Could you check a few things on this model? Use its own coordinates, in mm. A direction names the side the tool comes from. Give positions to 0.01 mm unless a question says otherwise; leave off trailing zeros. Write each loop counter-clockwise with the first axis right and the second up, starting at its lowest first coordinate (ties: lowest second). Pieces come first, ordered by that corner, then holes. Notation, with made-up numbers: (-3, 50) -> (14, 50) arc R26 cw to (14, 89) -> close; hole circle Ø11 at (62, 1). An arc over 180 degrees is marked (long way). One line per question, with ' | ' between items.
Autodesk Inventor part; units mm, degrees
ref_plane "YZ Plane" through (0, 0, 0) normal (1, 0, 0) x (0, 1, 0)
ref_plane "XZ Plane" through (0, 0, 0) normal (0, 1, 0) x (-1, 0, 0)
ref_plane "XY Plane" through (0, 0, 0) normal (0, 0, 1) x (1, 0, 0)
sketch "Sketch1" plane through (0, 0, 0) normal (0, 0, 1) x (1, 0, 0)
  line L0 (0, 3) -> (0, 18)
  line L1 (0, 18) -> (4, 18)
  line L2 (4, 18) -> (4, 15)
  line L3 (4, 15) -> (94, 15)
  line L4 (94, 15) -> (94, 18)
  line L5 (94, 18) -> (98, 18)
  line L6 (98, 18) -> (98, 12)
  line L7 (98, 12) -> (3, 12)
  line L8 (3, 12) -> (3, 3)
  line L9 (3, 0) -> (0, 0) construction
  line L10 (0, 3) -> (3, 3)
  dimension "d0" = 18
  dimension "d1" = 4
  dimension "d2" = 3
  dimension "d3" = 90
  dimension "d4" = 4
  dimension "d5" = 6
  dimension "d6" = 95
  dimension "d7" = 3
revolve "Revolution1" add sketch "Sketch1" angle 360 about axis through (3, 0, 0) along (-1, 0, 0)
properties part number "Filament Spool Holder"
Q1. Imagine slicing it at C-C on x = 50. Please give me the cut outline in (y, z).
Answer below:
outline: circle Ø30 at (0, 0); hole circle Ø24 at (0, 0)
Q2. If we mould it in two halves opening along Y, with no side actions, what happens to faces 4 (the cylindrical face through (49.84, -11.99, -0.53)), 5 (the cylindrical face through (49.63, -14.985, 0.66)), 6 (the flat face through (4, -4, -15))? For each: +Y half, -Y half, draft (parallel to the pull), parting line (faces both ways), or undercut.
Answer below:
face 4: undercut | face 5: parting line | face 6: draft
Q3. On a 3-axis mill with a long thin cutter (end or side, diameter ignored), from which of +Z, -Z, +X, -X, +Y, -Y can I reach the whole of each face in a straight line? I mean faces 1 (the flat face through (94, -4, -15)), 2 (the cylindrical face through (96.028, -2.343, 17.847)), 3 (the flat face through (3, 2.5, 2.5)). Say none if no direction works.
Answer below:
face 1: none | face 2: +X, -X | face 3: +X
Q4. Will these pins go through, and if not, where does the flat tip stop? pin 1 (3 mm diameter, centred on x = 63, z = -9.5, fed in from +Y); pin 2 (7 mm diameter, centred on y = 0, z = 0, fed in from +X); pin 3 (5 mm diameter, centred on x = 61.5, z = -14, fed in from -Y).
Answer below:
pin 1: stops at y = 12.69 | pin 2: stops at x = 3 | pin 3: stops at y = -9.63
Q5. Imagine slicing it at A-A on z = 0. Please give me the cut outline in (x, y).
Answer below:
outline: (0, -18) -> (4, -18) -> (4, -15) -> (94, -15) -> (94, -18) -> (98, -18) -> (98, -12) -> (3, -12) -> (3, -3) -> (0, -3) -> close; (0, 3) -> (3, 3) -> (3, 12) -> (98, 12) -> (98, 18) -> (94, 18) -> (94, 15) -> (4, 15) -> (4, 18) -> (0, 18) -> close
Q6. If I drill on line 1 along Y through (x, z) = (91.5, 0); line 2 along Y through (x, z) = (1, 0), over which ranges is the centre line in solid material (lowest first)?
Answer below:
line 1: y = -15 to -12, 12 to 15 | line 2: y = -18 to -3, 3 to 18
Q7. Imagine slicing it at D-D on y = 10. Please give me the cut outline in (x, z), and give its area (3 significant figures).
Answer below:
outline: (0, -14.97) -> (4, -14.97) -> (4, -11.18) -> (94, -11.18) -> (94, -14.97) -> (98, -14.97) -> (98, -6.63) -> (3, -6.63) -> (3, 6.63) -> (98, 6.63) -> (98, 14.97) -> (94, 14.97) -> (94, 11.18) -> (4, 11.18) -> (4, 14.97) -> (0, 14.97) -> close | area: 992 mm^2
